Check sheet for the modelled part. Datum: model origin and axes. Units: mm. Face numbers are marked on the shaded views. A direction names the side the tool comes from. Round coordinates to 2 decimals unless told otherwise and drop trailing zeros. Write each loop counter-clockwise with the first axis right and the second up, starting at its lowest first coordinate (ties: lowest second). Pieces come first, ordered by that corner, then holes.
Item 1: Set-up check for the marked faces 1 and 2: record each of +Z, -Z, +X, -X, +Y, -Y from which the full face is reachable in a straight line by a thin tool's end or side.
Item 2: Section check D-D, the plane y = -2. Record the cut outline in (x, z), plus the area to 3 significant figures.
Item 3: Material ranges on line 1 along Y through (x, z) = (16, 0); line 2 along X through (y, z) = (5.5, 0); line 3 along Z through (x, y) = (0, 4.25), recorded low to high.
Item 4: Depth check by flat-ended pin: pin 1 (8 mm diameter, centred on x = -17, z = 29.5, fed in from -Y); pin 2 (1.6 mm diameter, centred on x = 1, z = 0, fed in from +Y); pin 3 (3 mm diameter, centred on x = 12, y = 4.5, fed in from -Z). Enter the tip coordinate at first touch or a pass-through.
Item 5: Section check C-C, the plane y = 3.5. Record the cut outline in (x, z).
Item 6: Section check B-B, the plane z = 0. Record the cut outline in (x, y).
Item 7: Section check A-A, the plane x = 0. Record the cut outline in (y, z), plus the area to 3 significant figures.
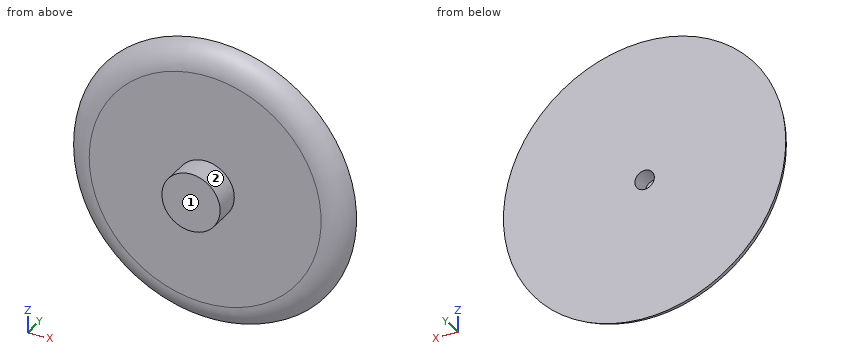
Solid Edge part; units mm, degrees
sketch "Sketch1" plane through (0, 0, 0) normal (0, 0, 1) x (1, 0, 0)
  line L0 (-37.5895, 1.7294) -> (-2.5895, 1.7294)
  line L1 (-2.5895, 1.7294) -> (-2.5895, 6.7294)
  line L2 (-2.5895, 6.7294) -> (-37.5895, 6.7294)
  line L3 (-37.5895, 6.7294) -> (-37.5895, 1.7294)
revolve "RevolvedProtrusion1" add sketch "Sketch1" angle 360 about axis through (0, 54, 0) along (0, -1, 0)
fillet "Round1" radius 7 1 edges at (-37.5895, 1.7294, 0)
sketch "Sketch2" plane through (0, 1.7294, 0) normal (0, -1, 0) x (1, 0, 0)
  circle A0 centre (0, 0) radius 7.7513
extrude "ExtrudedProtrusion_1" add sketch "Sketch2" along normal blind 6.9361
properties material "Aluminum Alloy:3.1255, AlCu4SiMg, EN-AW 2014"
Values found:
1. face 1: +Z, -Z, +X, -X, -Y
1. face 2: -Y
2. outline: circle Ø15.5 at (0, 0)
2. area: 189 mm2
3. line 1: y = 1.73 to 6.73
3. line 2: x = -37.09 to -2.59, 2.59 to 37.09
3. line 3: z = -36.26 to -2.59, 2.59 to 36.26
4. pin 1: stops at y = 1.73
4. pin 2: stops at y = 1.73
4. pin 3: stops at z = -35.5
5. outline: circle Ø71.07 at (0, 0); hole circle Ø5.18 at (0, 0)
6. outline: (-37.59, 6.73) arc R7 ccw to (-30.88, 1.73) - (-7.75, 1.73) - (-7.75, -5.21) - (7.75, -5.21) - (7.75, 1.73) - (30.88, 1.73) arc R7 ccw to (37.59, 6.73) - (2.59, 6.73) - (2.59, 1.73) - (-2.59, 1.73) - (-2.59, 6.73) - close
7. outline: (-5.21, -7.75) - (1.73, -7.75) - (1.73, -30.88) arc R7 ccw to (6.73, -37.59) - (6.73, -2.59) - (1.73, -2.59) - (1.73, 2.59) - (6.73, 2.59) - (6.73, 37.59) arc R7 ccw to (1.73, 30.88) - (1.73, 7.75) - (-5.21, 7.75) - close
7. area: 440 mm2
